The model under review builds one solid part; all positions refer to its coordinate system, in mm. A direction names the side the tool comes from. Round coordinates to 2 decimals unless told otherwise and drop trailing zeros. Write each loop counter-clockwise with the first axis right and the second up, starting at its lowest first coordinate (ties: lowest second). Pieces come first, ordered by that corner, then holes. Notation, with made-up numbers: (37, 30.25) - (61, 30.25) arc R29 ccw to (61, 69.25) - close; hole circle Ø3 at (51, 2.25). An arc over 180 degrees is marked (long way). Use one line per item in the form item = value.
Autodesk Inventor part; units mm, degrees
ref_plane "YZ Plane" through (0, 0, 0) normal (1, 0, 0) x (0, 1, 0)
ref_plane "XZ Plane" through (0, 0, 0) normal (0, 1, 0) x (-1, 0, 0)
ref_plane "XY Plane" through (0, 0, 0) normal (0, 0, 1) x (1, 0, 0)
sketch "スケッチ6" plane through (0, 0, 0) normal (0, 0, 1) x (1, 0, 0)
  point P0 (0, 0)
sketch "スケッチ7" plane through (0, 0, 0) normal (0, 0, 1) x (1, 0, 0)
  circle A0 centre (0, 0) radius 10
  circle A1 centre (0, 0) radius 6
  point P0 (0, 6)
  point P1 (-6, 0)
  point P2 (0, -6)
  point P3 (6, 0)
  dimension "d29" = 12
  dimension "d28" = 20
  dimension "d32" = 360
extrude "押し出し5" add sketch "スケッチ7" along normal blind 3 contours A0 | A1
sketch "スケッチ8" plane through (0, 0, 3) normal (0, 0, 1) x (1, 0, 0)
  circle A0 centre (0, 0) radius 6
  point P0 (0, 6)
  point P1 (-6, 0)
  point P2 (0, -6)
  point P3 (6, 0)
  dimension "d36" = 12
  dimension "d39" = 360
hole "穴2" at (0, 6, 3) at (-6, 0, 3) at (0, -6, 3) at (6, 0, 3) direction (0, 0, -1) diameter 1.5 end through all
sketch "スケッチ9" plane through (0, 0, 3) normal (0, 0, 1) x (1, 0, 0)
  circle A0 centre (0, 0) radius 3.5
  dimension "d48" = 7
extrude "押し出し6" add sketch "スケッチ9" along normal blind 6
properties part number "gear_01"
(1) The part is to be moulded in two halves that separate along X. For faces 1 (the cylindrical face through (-5.268, 0.163, 1.479)), 2 (the flat face through (0, 0, 0)), 3 (the cylindrical face through (-2.17, 9.76, 1.48)), say which applies: +X half, -X half, draft (parallel to the pull), parting line (faces both ways), or undercut.
Geometry results:
face_1 = undercut
face_2 = draft
face_3 = parting line
(2) Add section B-B on x = 0. Write out the cut boundary in (y, z).
Geometry results:
outline = (-10, 0) - (-6.75, 0) - (-6.75, 3) - (-10, 3) - close; (-5.25, 0) - (5.25, 0) - (5.25, 3) - (3.5, 3) - (3.5, 9) - (-3.5, 9) - (-3.5, 3) - (-5.25, 3) - close; (6.75, 0) - (10, 0) - (10, 3) - (6.75, 3) - close
(3) Insertion check: P1, Ø4, axis at y = -6, z = 1.5, coming from the +X side; P2, Ø1.5, axis at y = -5, z = 2, coming from the -X side; P3, Ø2, axis at x = 0, y = 6, coming from the +Z side. Each pin has a flat end and moves straight along its axis. Give the tip position at first contact, or say it passes through.
Geometry results:
P1 = 9.17
P2 = -9.05
P3 = 3
(4) To check wall thickness, follow L1, parallel to Y at x = 0, z = 0.9; L2, parallel to Z at x = -7.5, y = -4.5; L3, parallel to Y at x = -6.25, z = 0.5. State the ranges of each line that lie inside material, in increasing order.
Geometry results:
L1 = -10 to -6.75, -5.25 to 5.25, 6.75 to 10
L2 = 0 to 3
L3 = -7.81 to -0.71, 0.71 to 7.81
(5) Add section A-A on y = -6. Write out the cut boundary in (x, z), then the cut area to 3 significant figures.
Geometry results:
outline = (-8, 0) - (-0.75, 0) - (-0.75, 3) - (-8, 3) - close; (0.75, 0) - (8, 0) - (8, 3) - (0.75, 3) - close
area = 43.5 mm2
(6) Machinability: for faces 4 (the flat face through (0, 0, 9)), 5 (the flat face through (4, 0, 3)), which of the approach directions +Z, -Z, +X, -X, +Y, -Y give a long, thin tool a straight path to every point of the face, cutting with its end or side? Answer none if there is none.
Geometry results:
face_4 = +Z, +X, -X, +Y, -Y
face_5 = +Z
